Autodesk Inventor part; units mm, degrees
ref_plane "YZ Plane" through (0, 0, 0) normal (1, 0, 0) x (0, 1, 0)
ref_plane "XZ Plane" through (0, 0, 0) normal (0, 1, 0) x (-1, 0, 0)
ref_plane "XY Plane" through (0, 0, 0) normal (0, 0, 1) x (1, 0, 0)
sketch "Sketch2" plane through (0, 0, 0) normal (1, 0, 0) x (0, 1, 0)
  line L0 (0, 0) -> (17, 0)
  line L1 (17, 0) -> (17, -15)
  line L2 (17, -15) -> (0, -15)
  line L3 (0, -15) -> (0, 0)
  dimension "d4" = 17
  dimension "d5" = 15
extrude "Extrusion2" add sketch "Sketch2" along normal blind 157
sketch "Sketch3" plane through (157, 0, 0) normal (1, 0, 0) x (0, 0, -1)
  line L0 (0, 17) -> (0, 0)
  line L1 (0, 0) -> (15, 0)
  line L2 (15, 0) -> (15, 17)
  line L3 (2, 2) -> (13, 2)
  line L4 (13, 2) -> (13, 15)
  line L5 (13, 15) -> (2, 15)
  line L6 (2, 15) -> (2, 2)
  line L7 (2, 2) -> (13, 15) construction
  line L8 (13, 2) -> (2, 15) construction
  point P0 (7.5, 8.5)
  dimension "d9" = 11
  dimension "d10" = 13
extrude "Extrusion3" cut sketch "Sketch3" against normal through all
sketch "Sketch5" plane through (0, 0, -15) normal (0, 0, -1) x (-1, 0, 0)
  line L0 (0, 0) -> (-157, 0)
  line L1 (-157, 0) -> (0, 17)
  line L2 (-157, 0) -> (-157, 17)
  line L3 (0, 0) -> (-157, 17)
  circle A0 centre (-78.5, 8.5) radius 1.75
  dimension "d13" = 3.5
extrude "Extrusion4" cut sketch "Sketch5" against normal through all contours A0 L1 L3 | L3 L1 A0 | A0 L3 L1 | L3 A0 L1
fillet "Fillet1" radius 1 4 edges at (78.5, 2, -13) (78.5, 2, -2) (78.5, 15, -2) (78.5, 15, -13)
properties part number "caja perfil"
For this review, take the finished solid that the model builds, in its own axes (mm). A direction names the side the tool comes from. Give positions to 0.01 mm unless a question says otherwise; leave off trailing zeros. Write each loop counter-clockwise with the first axis right and the second up, starting at its lowest first coordinate (ties: lowest second). Pieces come first, ordered by that corner, then holes.
Item 1: Take a section at B-B (y = 8.5). Give the boundary of the cut face in (x, z).
Item 2: Insertion check: P1, Ø3, axis at x = 78.5, y = 8.5, coming from the +Z side. The pin has a flat end and moves straight along its axis. Give the tip position at first contact, or say it passes through.
Item 3: Wall thickness on probe 1 along Z at (x, y) = (96.5, 10.75); probe 2 along Y at (x, z) = (78.5, -1.5); probe 3 along Y at (x, z) = (106, -10): over which ranges is each line inside the solid? List them lowest first.
Item 4: Take a section at A-A (z = -6.5). Give the boundary of the cut face in (x, y), and give its area (3 significant figures).
Item 5: Take a section at C-C (x = 78.5). Give the boundary of the cut face in (y, z).
Item 6: Machinability: for faces 1 (the face through (76.831, 9.026, -14.014)), 2 (the face through (80, 11, -13)), which of the approach directions +Z, -Z, +X, -X, +Y, -Y give a long, thin tool a straight path to every point of the face, cutting with its end or side? Answer none if there is none.
Item 7: The part is to be moulded in two halves that separate along Y. For faces 3 (the face through (80, 15, -8)), 4 (the face through (77, 0, -8)), 5 (the face through (0, 8, -1)), 6 (the face through (77, 17, -7)), say which applies: +Y half, -Y half, draft (parallel to the pull), parting line (faces both ways), or undercut.
Established:
1. outline: (0, -15) - (76.75, -15) - (76.75, -13) - (0, -13) - close; (0, -2) - (76.75, -2) - (76.75, 0) - (0, 0) - close; (80.25, -15) - (157, -15) - (157, -13) - (80.25, -13) - close; (80.25, -2) - (157, -2) - (157, 0) - (80.25, 0) - close
2. P1: passes through
3. probe 1: z = -15 to -13, -2 to 0
3. probe 2: y = 0 to 6.75, 10.25 to 17
3. probe 3: y = 0 to 2, 15 to 17
4. outline: (0, 0) - (157, 0) - (157, 2) - (0, 2) - close; (0, 15) - (157, 15) - (157, 17) - (0, 17) - close
4. area: 628 mm2
5. outline: (0, -15) - (6.75, -15) - (6.75, -13) - (3, -13) arc R1 cw to (2, -12) - (2, -3) arc R1 cw to (3, -2) - (6.75, -2) - (6.75, 0) - (0, 0) - close; (10.25, -15) - (17, -15) - (17, 0) - (10.25, 0) - (10.25, -2) - (14, -2) arc R1 cw to (15, -3) - (15, -12) arc R1 cw to (14, -13) - (10.25, -13) - close
6. face 1: +Z, -Z
6. face 2: +X, -X
7. face 3: undercut
7. face 4: -Y half
7. face 5: draft
7. face 6: +Y half
